Geometry: see drawing. Coordinates: mm, zero at the bounding-box minimum. A direction names the side the tool comes from. Round coordinates to 2 decimals unless told otherwise and drop trailing zeros. Loops run counter-clockwise (first coordinate to the right, second up) from the corner with the lowest first, then second, coordinate; pieces in that order, holes last. Notation, with made-up numbers: (84.25, -16.5) - (100.25, -16.5) arc R28 cw to (100.25, 9.5) - close; hole circle Ø3 at (4, 32.5). An arc over 180 degrees is marked (long way). Return JSON: item names as keys, results as strings. Group by question number.
1. Material intervals for probe 1 along Y at (x, z) = (366.25, 50); probe 2 along X at (y, z) = (87, 5); probe 3 along Y at (x, z) = (73, 36), sorted ascending.
2. Section D-D on z = 61.5. Return loops of the section in (x, y).
3. Set-up query: the marked faces 5 and 6. Return all of +Z, -Z, +X, -X, +Y, -Y with unobstructed straight access to the full face (end or side cutting, diameter ignored); none if empty.
4. Section B-B on z = 41.5. Return loops of the section in (x, y), and give its area (3 significant figures).
5. Section C-C on z = 14.5. Return loops of the section in (x, y), and give its area (3 significant figures).
6. Section A-A on y = 88. Return loops of the section in (x, z).
7. Draft query along X for the marked faces 1, 2, 3 and 4. Return one class per face: +X half, -X half, draft (parallel to the pull), parting line (faces both ways), or undercut.
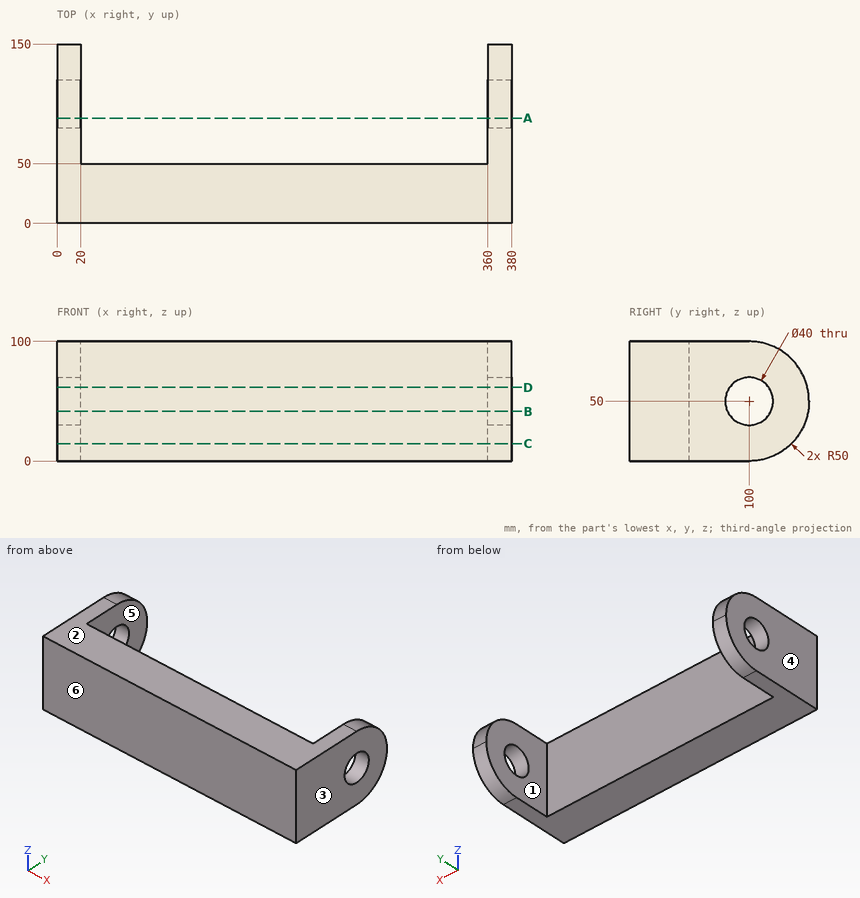
Taken from the geometry:
{
 "1": {"probe 1": "0 to 80, 120 to 150", "probe 2": "0 to 20, 360 to 380", "probe 3": "0 to 50"},
 "2": {"outline": "(0, 0) - (380, 0) - (380, 83.64) - (360, 83.64) - (360, 50) - (20, 50) - (20, 83.64) - (0, 83.64) - close; (0, 116.36) - (20, 116.36) - (20, 148.66) - (0, 148.66) - close; (360, 116.36) - (380, 116.36) - (380, 148.66) - (360, 148.66) - close"},
 "3": {"face 5": "+Z, -Z, +Y", "face 6": "+Z, -Z, +X, -X, -Y"},
 "4": {"outline": "(0, 0) - (380, 0) - (380, 81.9) - (360, 81.9) - (360, 50) - (20, 50) - (20, 81.9) - (0, 81.9) - close; (0, 118.1) - (20, 118.1) - (20, 149.27) - (0, 149.27) - close; (360, 118.1) - (380, 118.1) - (380, 149.27) - (360, 149.27) - close", "area": "21,500 mm2"},
 "5": {"outline": "(0, 0) - (380, 0) - (380, 135.21) - (360, 135.21) - (360, 50) - (20, 50) - (20, 135.21) - (0, 135.21) - close", "area": "22,400 mm2"},
 "6": {"outline": "(0, 0) - (20, 0) - (20, 34) - (0, 34) - close; (0, 66) - (20, 66) - (20, 100) - (0, 100) - close; (360, 0) - (380, 0) - (380, 34) - (360, 34) - close; (360, 66) - (380, 66) - (380, 100) - (360, 100) - close"},
 "7": {"face 1": "undercut", "face 2": "draft", "face 3": "+X half", "face 4": "-X half"}
}
